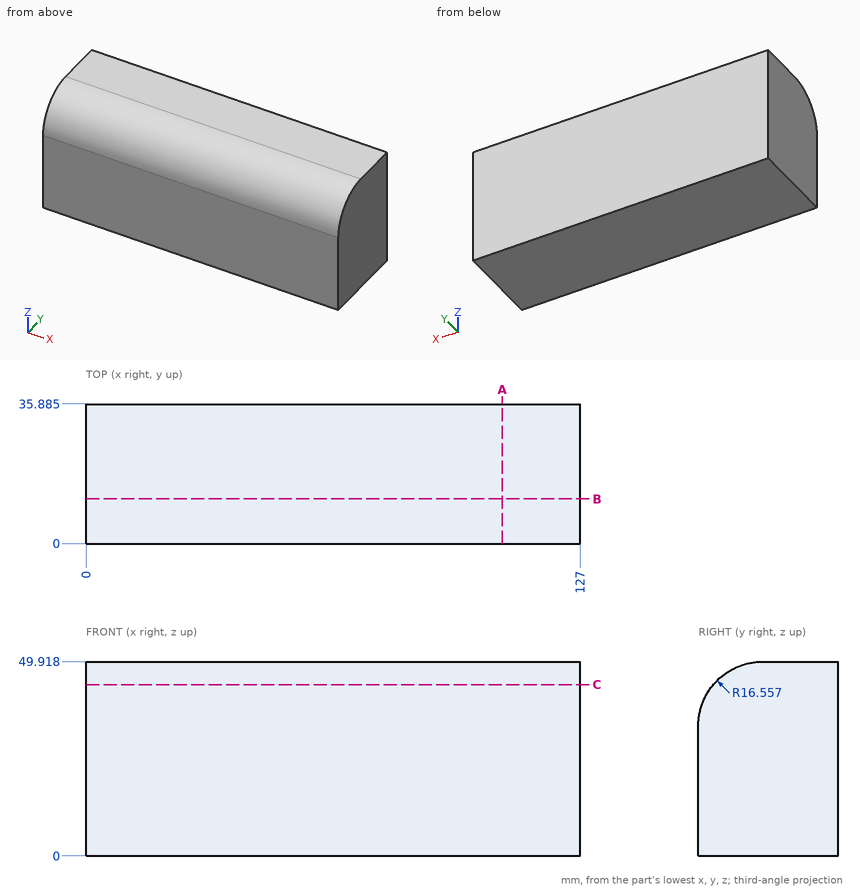
Input: dimensioned drawing with shaded views. Units: mm. Origin: part minimum x, y, z. Give positions to 0.01 mm unless a question says otherwise; leave off trailing zeros. Order: outer loops, then holes, each group sorted by start corner. A loop starts at its lowest first (then second) coordinate and runs counter-clockwise, first axis right, second up.
(1) Section query B-B (y = 11.5). Return the cut outline in (x, z), plus the area to 3 significant figures.
(2) Section query A-A (x = 107). Return the cut outline in (y, z) (1 decimal), plus the area to 3 significant figures.
(3) Material intervals for line 1 along Z through (x, y) = (64.5, 15) (1 decimal); line 2 along Y through (x, z) = (65, 42) (1 decimal); line 3 along Y through (x, z) = (57, 34.5) (1 decimal), sorted ascending.
(4) Contact query for flat-ended pins moving along their axis: P1, Ø2, axis at x = 29.5, z = 36.5, coming from the -Y side; P2, Ø4, axis at x = 38, y = 6.5, coming from the +Z side (1 decimal). Output: stop coordinate, or through.
(5) Section query C-C (z = 44). Return the cut outline in (x, y) (1 decimal).
Outcome:
1. outline: (0, 0) - (127, 0) - (127, 49.13) - (0, 49.13) - close
1. area: 6,240 mm2
2. outline: (0, 0) - (35.9, 0) - (35.9, 49.9) - (16.6, 49.9) arc R16.6 ccw to (0, 33.4) - close
2. area: 1,730 mm2
3. line 1: z = 0 to 49.8
3. line 2: y = 2.4 to 35.9
3. line 3: y = 0 to 35.9
4. P1: stops at y = 0.14
4. P2: stops at z = 47.8
5. outline: (0, 3.9) - (127, 3.9) - (127, 35.9) - (0, 35.9) - close
